```python
from build123d import *

# Parameters (mm, degrees)
F0_W     = 127
F0_H     = 63.5
F1_DEPTH = 12.7
F2_R     = 12.7
F3_DEPTH = 44.45
F5_DEPTH = 57.15
F7_R     = 5.08
F8_DEPTH = 25.4


with BuildPart() as f1:
    # F0 (on Front) → F1 (new body)
    with BuildSketch(Plane.XZ):
        Rectangle(F0_W, F0_H)
    extrude(amount=F1_DEPTH)

    # F2 (on face) → F3 (join)
    with BuildSketch(Plane.XZ.offset(12.7)):
        with BuildLine():
            Line((-63.5, -19.05), (-63.5, -31.75))
            Line((-63.5, -31.75), (63.5, -31.75))
            Line((63.5, -31.75), (63.5, -19.05))
            Line((63.5, -19.05), (47.625, -19.05))
            Line((47.625, -19.05), (21.0934256055, 20.5001730104))
            ThreePointArc((21.0934256055, 20.5001730104), (11.9529411765, 28.7617647059), (0, 31.75))
            ThreePointArc((0, 31.75), (-11.9529411765, 28.7617647059), (-21.0934256055, 20.5001730104))
            Line((-21.0934256055, 20.5001730104), (-47.625, -19.05))
            Line((-47.625, -19.05), (-63.5, -19.05))
        make_face()
        with Locations((0, 6.35)):
            Circle(F2_R, mode=Mode.SUBTRACT)
    extrude(amount=F3_DEPTH)

    # F4 (on Front) → F5 (join)
    with BuildSketch(Plane.XZ):
        Polygon((12.7, -31.75), (-12.7, -31.75), (-12.7, -40.64), (-31.75, -40.64), (-31.75, -53.34), (31.75, -53.34), (31.75, -40.64), (12.7, -40.64), align=None)
    extrude(amount=F5_DEPTH)

    # F7 (on offset) → F8 (cut)
    with BuildSketch(Plane.XY.offset(6.35)):
        with Locations((0, -34.925)):
            Circle(F7_R)
    extrude(amount=F8_DEPTH, mode=Mode.SUBTRACT)


solid = f1.part
```
Here's how the part is built. I have some questions about the finished solid (model axes, mm). A direction names the side the tool comes from. Coordinates: 2 decimals unless noted, no trailing zeros. Order: outer loops, then holes, each group sorted by start corner. A loop starts at its lowest first (then second) coordinate and runs counter-clockwise, first axis right, second up. Notation, with made-up numbers: (-33.5, -20.5) - (-18.5, -20.5) arc R22 cw to (-18.5, 8.5) - close; hole circle Ø9 at (-39.5, 77.5). An arc over 180 degrees is marked (long way). One line per question, with ' | ' between items.
(1) Suppose I cut it at B-B on y = -24. List the corners of the cut face in (x, z) for me (3 decimals).
Report:
outline: (-63.5, -31.75) - (-12.7, -31.75) - (-12.7, -40.64) - (-31.75, -40.64) - (-31.75, -53.34) - (31.75, -53.34) - (31.75, -40.64) - (12.7, -40.64) - (12.7, -31.75) - (63.5, -31.75) - (63.5, -19.05) - (47.625, -19.05) - (21.093, 20.5) arc R25.4 ccw to (-21.093, 20.5) - (-47.625, -19.05) - (-63.5, -19.05) - close; hole circle Ø25.4 at (0, 6.35)
(2) Suppose I cut it at D-D on z = -2.5. List the corners of the cut face in (x, y) for me, and give its area (3 significant figures).
Report:
outline: (-63.5, -12.7) - (-36.52, -12.7) - (-36.52, -57.15) - (-9.11, -57.15) - (-9.11, -12.7) - (9.11, -12.7) - (9.11, -57.15) - (36.52, -57.15) - (36.52, -12.7) - (63.5, -12.7) - (63.5, 0) - (-63.5, 0) - close | area: 4,050 mm2
(3) Will these pins go through, and if not, where does the flat tip stop? pin 1 (10 mm diameter, centred on y = -38, z = 15.5, fed in from +X); pin 2 (6 mm diameter, centred on x = 28, z = -32.5, fed in from +Y); pin 3 (7.5 mm diameter, centred on x = 1.5, z = 4, fed in from -Y); pin 4 (4.5 mm diameter, centred on y = -27, z = -34.5, fed in from -X).
Report:
pin 1: stops at x = 27.8 | pin 2: stops at y = 0 | pin 3: stops at y = -12.7 | pin 4: stops at x = -12.7
(4) Suppose I cut it at A-A on x = 18. List the corners of the cut face in (y, z) for me, and give its area (3 significant figures).
Report:
outline: (-57.15, -53.34) - (0, -53.34) - (0, -40.64) - (-57.15, -40.64) - close; (-57.15, -31.75) - (0, -31.75) - (0, 31.75) - (-12.7, 31.75) - (-12.7, 24.27) - (-57.15, 24.27) - close | area: 4,020 mm2
(5) If we mould it in two halves opening along Z, with no side actions, what happens to faces 4 (the flat face through (-12.7, -28, -36)), 5 (the flat face through (-34.173, -34.614, 1.002)), 6 (the flat face through (-63.5, -9, -14))? For each: pulls with the +Z half, pulls with the -Z half, needs draft (parallel to the pull), parting line crosses it, or undercut.
Report:
face 4: undercut | face 5: pulls with the +Z half | face 6: needs draft
(6) Suppose I cut it at C-C on z = 25.5. List the corners of the cut face in (x, y) for me (3 decimals), and give its area (3 significant figures).
Report:
outline: (-63.5, -12.7) - (-16.686, -12.7) - (-16.686, -57.15) - (16.686, -57.15) - (16.686, -12.7) - (63.5, -12.7) - (63.5, 0) - (-63.5, 0) - close; hole circle Ø10.16 at (0, -34.925) | area: 3,020 mm2
(7) For faces 1 (the flat face through (0, -12.7, 7)), 2 (the flat face through (12.7, -28, -36)), 3 (the flat face through (-46, -12.7, 12)), which set-ups out of +Z, -Z, +X, -X, +Y, -Y let a thin tool reach every point of the face, with its end or its side?
Report:
face 1: -Y | face 2: +X, +Y, -Y | face 3: +Z, -X, -Y
(8) If I drill on L1, parallel to Z at x = 0, y = -26.5; L2, parallel to Y at x = 0, z = 22 (3 decimals); L3, parallel to Z at x = 57, y = -17, over which ranges is the centre line in solid material (lowest first)?
Report:
L1: z = -53.34 to -6.35, 19.05 to 31.75 | L2: y = -57.15 to -40.005, -29.845 to 0 | L3: z = -31.75 to -19.05
